Could you check a few things on this drawing? It's one solid part, dimensions in mm from its lowest x, y, z. A direction names the side the tool comes from. Round coordinates to 2 decimals unless told otherwise and drop trailing zeros. Loops run counter-clockwise (first coordinate to the right, second up) from the corner with the lowest first, then second, coordinate; pieces in that order, holes last. Notation, with made-up numbers: (8, 78.5) -> (67, 78.5) arc R6 cw to (67, 88.5) -> close; hole circle Ø8 at (81.25, 45). An arc over 180 degrees is marked (long way). Use one line per item in the form item = value. Start each with the question number.
Item 1: If we section it at C-C (z = 1243): Write out the boundary of the cut face in (x, y), then the cut area to 3 significant figures.
Item 2: For the marked faces 1 and 2, which set-ups out of +Z, -Z, +X, -X, +Y, -Y let a thin tool reach every point of the face, with its end or its side?
Item 3: If we section it at B-B (x = 530.5): Write out the boundary of the cut face in (y, z).
Item 4: I'm going to push a flat-ended pin straight in: pin 1 Ø6 at (x, z) = (167, 234) entering from -Y. Where does the tip first touch, or does it pass through?
Item 5: Thinking about a two-plate mould opening in Z: for the marked faces 3, 4, 5 and 6, which applies, released by +Z, released by -Z, zero draft, split by the parting line, or undercut?
Item 6: If I drill on L1, parallel to Z at x = 468, y = 72.5; L2, parallel to X at y = 57, z = 1292.5; L3, parallel to Y at x = 344.5, z = 110.5, over which ranges is the centre line in solid material (lowest first)? Write a range as [from, to].
Item 7: If we section it at A-A (y = 216.5): Write out the boundary of the cut face in (x, z).
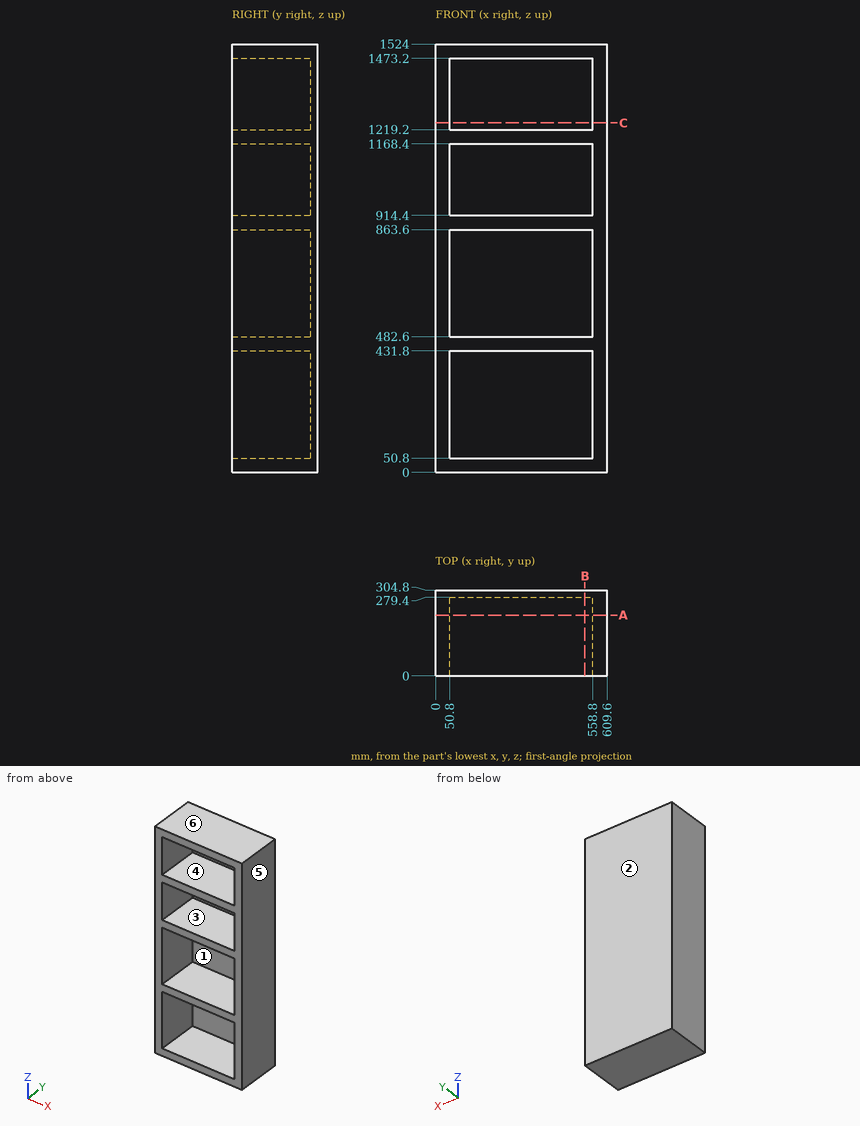
Values found:
q1.outline = (0, 0) -> (50.8, 0) -> (50.8, 279.4) -> (558.8, 279.4) -> (558.8, 0) -> (609.6, 0) -> (609.6, 304.8) -> (0, 304.8) -> close
q1.area = 43,900 mm2
q2.face_1 = -Y
q2.face_2 = +Z, -Z, +X, -X, +Y
q3.outline = (0, 0) -> (304.8, 0) -> (304.8, 1524) -> (0, 1524) -> (0, 1473.2) -> (279.4, 1473.2) -> (279.4, 1219.2) -> (0, 1219.2) -> (0, 1168.4) -> (279.4, 1168.4) -> (279.4, 914.4) -> (0, 914.4) -> (0, 863.6) -> (279.4, 863.6) -> (279.4, 482.6) -> (0, 482.6) -> (0, 431.8) -> (279.4, 431.8) -> (279.4, 50.8) -> (0, 50.8) -> close
q4.pin_1 = 279.4
q5.face_3 = undercut
q5.face_4 = undercut
q5.face_5 = zero draft
q5.face_6 = released by +Z
q6.L1 = [0, 50.8], [431.8, 482.6], [863.6, 914.4], [1168.4, 1219.2], [1473.2, 1524]
q6.L2 = [0, 50.8], [558.8, 609.6]
q6.L3 = [279.4, 304.8]
q7.outline = (0, 0) -> (609.6, 0) -> (609.6, 1524) -> (0, 1524) -> close; hole (50.8, 50.8) -> (558.8, 50.8) -> (558.8, 431.8) -> (50.8, 431.8) -> close; hole (50.8, 482.6) -> (558.8, 482.6) -> (558.8, 863.6) -> (50.8, 863.6) -> close; hole (50.8, 914.4) -> (558.8, 914.4) -> (558.8, 1168.4) -> (50.8, 1168.4) -> close; hole (50.8, 1219.2) -> (558.8, 1219.2) -> (558.8, 1473.2) -> (50.8, 1473.2) -> close
